Could you check a few things on this model? Use its own coordinates, in mm. Face numbers are marked on the shaded views. A direction names the side the tool comes from. Coordinates: 2 decimals unless noted, no trailing zeros. Loops run counter-clockwise (first coordinate to the right, second up) from the corner with the lowest first, then second, coordinate; pieces in that order, holes last. Notation, with made-up numbers: (18.25, 24) -> (25.25, 24) arc R18 ccw to (25.25, 50) -> close; hole circle Ø7 at (42.5, 20). An arc over 180 degrees is marked (long way). One line per question, with ' | ' between items. Start each with the question number.
(1) If I drill on line 1 along X through (y, z) = (1, 5.75); line 2 along X through (y, z) = (-5.5, 4); line 3 along X through (y, z) = (-2, 1), over which ranges is the centre line in solid material (lowest first)?
(2) Suppose I cut it at B-B (x = -34). Please give me the cut outline in (y, z), plus the area to 3 significant figures.
(3) Suppose I cut it at A-A (y = -2.5). Please give me the cut outline in (x, z).
(4) Which directions (+Z, -Z, +X, -X, +Y, -Y) give clear straight access to the entire face, cutting with the end or side of a thin tool? Please do the marked faces 1 and 2.
(5) I'm going to push flat-ended pins straight in: pin 1 Ø2 at (x, z) = (-30, 3.5) entering from +Y; pin 2 Ø2.5 at (x, y) = (-49.15, 0.88) entering from +Z; pin 3 Ø2 at (x, z) = (-17.5, 3.5) entering from -Y. Where does each tip first touch, or does it pass through?
Autodesk Inventor part; units mm, degrees
ref_plane "YZ Plane" through (0, 0, 0) normal (1, 0, 0) x (0, 1, 0)
ref_plane "XZ Plane" through (0, 0, 0) normal (0, 1, 0) x (-1, 0, 0)
ref_plane "XY Plane" through (0, 0, 0) normal (0, 0, 1) x (1, 0, 0)
sketch "Náčrt1" plane through (0, 0, 0) normal (0, 0, 1) x (1, 0, 0)
  line L0 (-46.6467, 2.3751) -> (53.3533, 2.3751)
  line L1 (53.3533, 2.3751) -> (53.3533, -4.6249)
  line L2 (53.3533, -4.6249) -> (-46.6467, -4.6249)
  line L3 (-46.6467, -4.6249) -> (-46.6467, 2.3751)
  line L4 (-46.6467, 4.3751) -> (-52.6467, 4.3751)
  line L5 (-52.6467, 4.3751) -> (-52.6467, -6.6249)
  line L6 (-46.6467, -6.6249) -> (-46.6467, 4.3751)
  line L7 (-50.6467, 2.3751) -> (-48.6467, 2.3751)
  line L8 (-48.6467, 2.3751) -> (-48.6467, -6.6249)
  line L9 (-50.6467, -6.6249) -> (-50.6467, 2.3751)
  line L10 (-52.6467, -6.6249) -> (-50.6467, -6.6249)
  line L11 (-48.6467, -6.6249) -> (-46.6467, -6.6249)
  line L12 (53.3533, 4.3751) -> (59.3533, 4.3751)
  line L13 (59.3533, 4.3751) -> (59.3533, -6.6249)
  line L14 (53.3533, -6.6249) -> (53.3533, 4.3751)
  line L15 (57.3533, -6.6249) -> (57.3533, 1.5943)
  line L16 (57.3533, 1.5943) -> (55.3533, 1.5943)
  line L17 (55.3533, 1.5943) -> (55.3533, -6.6249)
  line L18 (59.3533, -6.6249) -> (57.3533, -6.6249)
  line L19 (55.3533, -6.6249) -> (53.3533, -6.6249)
  point P0 (0, 0)
  point P1 (-47.6467, -6.6249)
  point P2 (56.3533, 4.3751)
  point P3 (55.3533, -2.5153)
  point P4 (54.3533, -6.6249)
  dimension "d0" = 100
  dimension "d1" = 7
  dimension "d2" = 2
  dimension "d4" = 6
  dimension "d5" = 2
  dimension "d6" = 0
  dimension "d7" = 2
  dimension "d8" = 2
  dimension "d9" = 2
  dimension "d10" = 2
  dimension "d11" = 6
  dimension "d12" = 0
  dimension "d14" = 2
  dimension "d15" = 2
  dimension "d16" = 2
extrude "Vysunutí1" add sketch "Náčrt1" along normal blind 7
fillet "Zaoblení1" radius 1 3 edges at (-46.6467, 4.3751, 3.5) (-46.6467, 2.3751, 3.5) (-52.6467, 4.3751, 3.5)
fillet "Zaoblení2" radius 1 3 edges at (53.3533, 2.3751, 3.5) (53.3533, 4.3751, 3.5) (59.3533, 4.3751, 3.5)
fillet "Zaoblení3" radius 1 5 edges at (-46.6467, -4.6249, 3.5) (-46.6467, -6.6249, 3.5) (-48.6467, -6.6249, 3.5) (-50.6467, -6.6249, 3.5) (-52.6467, -6.6249, 3.5)
fillet "Zaoblení4" radius 1 5 edges at (53.3533, -6.6249, 3.5) (53.3533, -4.6249, 3.5) (55.3533, -6.6249, 3.5) (57.3533, -6.6249, 3.5) (59.3533, -6.6249, 3.5)
fillet "Zaoblení5" radius 1 4 edges at (-50.6467, 2.3751, 3.5) (-48.6467, 2.3751, 3.5) (55.3533, 1.5943, 3.5) (57.3533, 1.5943, 3.5)
sketch "Náčrt2" plane through (0, 0, 7) normal (0, 0, 1) x (1, 0, 0)
  circle A0 centre (-49.1467, 0.8751) radius 2
  line L0 (-52.6467, 3.3751) -> (-52.6467, -5.6249)
  line L1 (-47.6467, 4.3751) -> (-51.6467, 4.3751)
  circle A1 centre (55.8533, 0.8751) radius 1.75
  line L2 (59.3533, -5.6249) -> (59.3533, 3.3751)
  line L3 (58.3533, 4.3751) -> (54.3533, 4.3751)
  point P0 (0, 0)
  dimension "d24" = 4
  dimension "d25" = 3.5
  dimension "d26" = 3.5
  dimension "d27" = 3.5
  dimension "d28" = 3.5
  dimension "d29" = 3.5
extrude "Vysunutí2" cut sketch "Náčrt2" against normal through all
properties part number "rozpěrka"
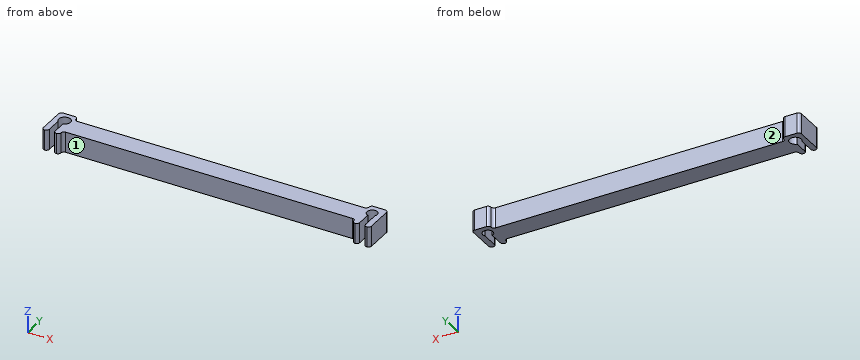
Checks:
1) line 1: x = -52.65 to -51.14, -47.15 to 54.11, 57.6 to 59.35 | line 2: x = -52.65 to -50.65, -48.65 to -46.64, 53.35 to 55.35, 57.35 to 59.35 | line 3: x = -52.65 to -50.65, -48.65 to 55.35, 57.35 to 59.35
2) outline: (-4.62, 0) -> (2.38, 0) -> (2.38, 7) -> (-4.62, 7) -> close | area: 49.0 mm^2
3) outline: (-52.65, 0) -> (-50.65, 0) -> (-50.65, 7) -> (-52.65, 7) -> close; (-48.65, 0) -> (55.35, 0) -> (55.35, 7) -> (-48.65, 7) -> close; (57.35, 0) -> (59.35, 0) -> (59.35, 7) -> (57.35, 7) -> close
4) face 1: +Z, -Z, -Y | face 2: +Z, -Z, +Y
5) pin 1: stops at y = 2.38 | pin 2: passes through | pin 3: stops at y = -4.62
